Could you check a few things on this model? Use its own coordinates, in mm. A direction names the side the tool comes from. Give positions to 0.01 mm unless a question says otherwise; leave off trailing zeros. Order: outer loops, then holes, each group sorted by start corner. A loop starts at its lowest first (then second) coordinate and runs counter-clockwise, first axis right, second up.
from build123d import *

# Parameters (mm, degrees)
BOSS_EXTRUDE1_DEPTH = 1.62
CHAMFER1_SIZE       = 0.5


with BuildPart() as part:
    # Sketch1 → Boss-Extrude1 (new body)
    with BuildSketch(Plane(origin=(0, 0, 0), x_dir=(1, 0, 0), z_dir=(0, 1, 0))):
        with BuildLine():
            ThreePointArc((17.5, 3), (20.5, 0), (17.5, -3))
            Line((17.5, -3), (-17.5, -3))
            Line((-17.5, -3), (-17.5, -10))
            Line((-17.5, -10), (42.5, -10))
            Line((42.5, -10), (42.5, 10))
            Line((42.5, 10), (-17.5, 10))
            Line((-17.5, 10), (-17.5, 3))
            Line((-17.5, 3), (17.5, 3))
        make_face()
    extrude(amount=BOSS_EXTRUDE1_DEPTH)

    # Chamfer1
    chamfer1_edges = [part.edges().sort_by_distance(p)[0] for p in [
        (-17.5, 0, -6.5),
        (12.5, 0, -10),
        (42.5, 0, 0),
        (12.5, 0, 10),
        (-17.5, 0, 6.5),
        (0, 0, 3),
        (20.5, 0, 0),
        (0, 0, -3),
    ]]
    chamfer(chamfer1_edges, length=CHAMFER1_SIZE)


solid = part.part
Item 1: We'd pull the mould along Z, two halves only. Please class faces 1 (the flat face through (13, 1, -10)), 2 (the cylindrical face through (20.5, 1.1, -0.1)), 3 (the flat face through (12, 1.62, -5)): +Z half, -Z half, draft (parallel to the pull), parting line (faces both ways), or undercut.
Findings:
face 1: -Z half
face 2: undercut
face 3: draft
Item 2: Please list where these lines run through material, in increasing order: line 1 along Z through (x, y) = (17.5, 0.65); line 2 along Z through (x, y) = (10.5, 0.1); line 3 along Z through (x, y) = (25.5, 0.15).
Findings:
line 1: z = -10 to -3, 3 to 10
line 2: z = -9.6 to -3.4, 3.4 to 9.6
line 3: z = -9.65 to 9.65
Item 3: Imagine slicing it at B-B on y = 1.1. List the corners of the cut face in (x, z) for me, then the cut area to 3 significant figures.
Findings:
outline: (-17.5, -10) - (42.5, -10) - (42.5, 10) - (-17.5, 10) - (-17.5, 3) - (17.5, 3) arc R3 cw to (17.5, -3) - (-17.5, -3) - close
area: 976 mm2
Item 4: For faces 4 (the flat face through (0, 1, 3)), 5 (the conical face through (20.64, 0.36, -0.07)), which set-ups out of +Z, -Z, +X, -X, +Y, -Y let a thin tool reach every point of the face, with its end or its side?
Findings:
face 4: -X, +Y, -Y
face 5: -X, -Y
Item 5: Imagine slicing it at C-C on z = 0. List the corners of the cut face in (x, y) for me, then the cut area to 3 significant figures.
Findings:
outline: (20.5, 0.5) - (21, 0) - (42, 0) - (42.5, 0.5) - (42.5, 1.62) - (20.5, 1.62) - close
area: 35.4 mm2
Item 6: Imagine slicing it at A-A on x = 11. List the corners of the cut face in (y, z) for me, then the cut area to 3 significant figures.
Findings:
outline: (0, -9.5) - (0.5, -10) - (1.62, -10) - (1.62, -3) - (0.5, -3) - (0, -3.5) - close; (0, 3.5) - (0.5, 3) - (1.62, 3) - (1.62, 10) - (0.5, 10) - (0, 9.5) - close
area: 22.2 mm2
